For this review, take the finished solid that the model builds, in its own axes (mm). A direction names the side the tool comes from. Give positions to 0.01 mm unless a question says otherwise; leave off trailing zeros. Order: outer loops, then holes, each group sorted by start corner. A loop starts at its lowest first (then second) coordinate and runs counter-clockwise, first axis right, second up. Notation, with made-up numbers: (35.5, 32) -> (61.5, 32) arc R27 cw to (61.5, 49) -> close; hole circle Ø1 at (73.5, -25). An arc over 180 degrees is marked (long way). Return JSON: item names as keys, results as strings. Group by question number.
1) Insertion check: P1, Ø3.5, axis at x = -19.5, y = 8.5, coming from the +Z side (3 decimals); P2, Ø1, axis at x = 89.5, y = 2, coming from the -Z side (3 decimals); P3, Ø1, axis at y = 1.5, z = 42.5, coming from the +X side. Each pin has a flat end and moves straight along its axis. Give the tip position at first contact, or say it passes through.
2) Add section A-A (y = 6.25). Give the boundary of the cut face in (x, z) (3 decimals), then the cut area to 3 significant figures.
3) To check wall thickness, follow line 1 along Z through (x, y) = (-49, 6.75) (3 decimals); line 2 along Z through (x, y) = (65, 4.75) (3 decimals); line 3 along Z through (x, y) = (24.5, 7.75) (3 decimals). State the ranges of each line that lie inside material, in increasing order.
4) Add section C-C (z = 12.5). Give the boundary of the cut face in (x, y) (3 decimals).
5) Add section B-B (x = -17). Give the boundary of the cut face in (y, z) (3 decimals), then the cut area to 3 significant figures.
6) Add section D-D (x = 60.5). Give the boundary of the cut face in (y, z) (3 decimals), then the cut area to 3 significant figures.
7) For faces 1 (the face through (79.375, 6, -40)), 2 (the face through (-0.745, 7.727, -29.738)), 3 (the face through (82.55, 2, -43)), 4 (the face through (87, 2, 10.16)), list the 3-axis set-ups (+Z, -Z, +X, -X, +Y, -Y) from which the entire face can be reached by the end or side of a thin tool; tool diameter is ignored.
8) The part is to be moulded in two halves that separate along Z. For faces 5 (the face through (89, 2, 41.275)), 6 (the face through (1, 9.525, 40)), 7 (the face through (57.15, 9, 0)), say which applies: released by +Z, released by -Z, zero draft, split by the parting line, or undercut.
from build123d import *

# Parameters (mm, degrees)
SKETCH1_W           = 165.1
SKETCH1_H           = 88.9
BOSS_EXTRUDE1_DEPTH = 3.175
SKETCH3_W           = 82.55
SKETCH3_H           = 3.175
BOSS_EXTRUDE3_DEPTH = 12.7
SKETCH6_W           = 19.05
SKETCH6_H           = 3.175
CUT_EXTRUDE1_DEPTH  = 16.002
SKETCH8_W           = 154.94
SKETCH8_H           = 3.437080139
BOSS_EXTRUDE4_DEPTH = 6.35
SKETCH9_W           = 114.3
SKETCH9_H           = 69.85
BOSS_EXTRUDE5_DEPTH = 15.24
SKETCH12_W          = 88.9
SKETCH12_H          = 50.8
CUT_EXTRUDE2_DEPTH  = 15.24
CUT_EXTRUDE2_DRAFT  = 30


with BuildPart() as part:
    # Sketch1 → Boss-Extrude1 (new body)
    with BuildSketch(Plane(origin=(0, 0, 0), x_dir=(1, 0, 0), z_dir=(0, 1, 0))):
        Rectangle(SKETCH1_W, SKETCH1_H)
    extrude(amount=BOSS_EXTRUDE1_DEPTH)

    # Sketch3 → Boss-Extrude3 (add)
    with BuildSketch(Plane(origin=(82.55, 0, 0), x_dir=(0, 0, -1), z_dir=(1, 0, 0))):
        with Locations((0, 1.5875)):
            Rectangle(SKETCH3_W, SKETCH3_H)
    extrude(amount=BOSS_EXTRUDE3_DEPTH)

    # Sketch6 → Cut-Extrude1 (cut)
    with BuildSketch(Plane(origin=(95.25, 0, 0), x_dir=(0, 0, -1), z_dir=(1, 0, 0))):
        with Locations((-0.635, 1.5875)):
            Rectangle(SKETCH6_W, SKETCH6_H)
    extrude(amount=-CUT_EXTRUDE1_DEPTH, mode=Mode.SUBTRACT)

    # Sketch8 → Boss-Extrude4 (add)
    with BuildSketch(Plane(origin=(0, 3.175, 0), x_dir=(1, 0, 0), z_dir=(0, 1, 0))):
        with Locations((1.905, -39.556459931)):
            Rectangle(SKETCH8_W, SKETCH8_H)
        with Locations((1.905, 39.556459931)):
            Rectangle(SKETCH8_W, SKETCH8_H)
    extrude(amount=BOSS_EXTRUDE4_DEPTH)

    # Sketch9 → Boss-Extrude5 (add)
    with BuildSketch(Plane(origin=(0, 0, 0), x_dir=(1, 0, 0), z_dir=(0, 1, 0))):
        Rectangle(SKETCH9_W, SKETCH9_H)
    extrude(amount=BOSS_EXTRUDE5_DEPTH)


with BuildPart() as cut_extrude2_tool:
    # Sketch12 → Cut-Extrude2 (with draft: the straight prism first)
    with BuildSketch(Plane(origin=(0, 15.24, 0), x_dir=(1, 0, 0), z_dir=(0, 1, 0))):
        Rectangle(SKETCH12_W, SKETCH12_H)
    extrude(amount=-CUT_EXTRUDE2_DEPTH)
    # Cut-Extrude2: the draft: its side faces are tilted about the plane it starts from
    cut_extrude2_sides = [cut_extrude2_tool.faces().sort_by_distance(p)[0] for p in [
        (-44.45, 7.62, 0),
        (0, 7.62, 25.4),
        (44.45, 7.62, 0),
        (0, 7.62, -25.4),
    ]]
    draft(cut_extrude2_sides, Plane(origin=(0, 15.24, 0), x_dir=(1, 0, 0), z_dir=(0, 1, 0)), CUT_EXTRUDE2_DRAFT)


with BuildPart() as part_1:
    add(part.part)

    # Cut-Extrude2: cut by cut_extrude2_tool
    add(cut_extrude2_tool.part, mode=Mode.SUBTRACT)


solid = part_1.part
Evaluation:
{
 "1": {"P1": "z = 41.275", "P2": "z = -41.275", "P3": "x = 82.55"},
 "2": {"outline": "(-75.565, -41.275) -> (79.375, -41.275) -> (79.375, -37.838) -> (-75.565, -37.838) -> close; (-75.565, 37.838) -> (79.375, 37.838) -> (79.375, 41.275) -> (-75.565, 41.275) -> close; (-57.15, -34.925) -> (57.15, -34.925) -> (57.15, 34.925) -> (-57.15, 34.925) -> close; hole (-49.64, -30.59) -> (49.64, -30.59) -> (49.64, 30.59) -> (-49.64, 30.59) -> close", "area": "2,970 mm^2"},
 "3": {"line 1": "-41.275 to -37.838, -34.925 to -30.302, 30.302 to 34.925, 37.838 to 41.275", "line 2": "-41.275 to -37.838, 37.838 to 41.275", "line 3": "-41.275 to -37.838, -34.925 to -29.724, 29.724 to 34.925, 37.838 to 41.275"},
 "4": {"outline": "(-82.55, 0) -> (-53.249, 0) -> (-44.45, 15.24) -> (-57.15, 15.24) -> (-57.15, 3.175) -> (-82.55, 3.175) -> close; (44.45, 15.24) -> (53.249, 0) -> (95.25, 0) -> (95.25, 3.175) -> (57.15, 3.175) -> (57.15, 15.24) -> close"},
 "5": {"outline": "(0, -44.45) -> (3.175, -44.45) -> (3.175, -41.275) -> (9.525, -41.275) -> (9.525, -37.838) -> (3.175, -37.838) -> (3.175, -34.925) -> (15.24, -34.925) -> (15.24, -25.4) -> (0, -34.199) -> close; (0, 34.199) -> (15.24, 25.4) -> (15.24, 34.925) -> (3.175, 34.925) -> (3.175, 37.838) -> (9.525, 37.838) -> (9.525, 41.275) -> (3.175, 41.275) -> (3.175, 44.45) -> (0, 44.45) -> close", "area": "260 mm^2"},
 "6": {"outline": "(0, -44.45) -> (3.175, -44.45) -> (3.175, -41.275) -> (9.525, -41.275) -> (9.525, -37.838) -> (3.175, -37.838) -> (3.175, 37.838) -> (9.525, 37.838) -> (9.525, 41.275) -> (3.175, 41.275) -> (3.175, 44.45) -> (0, 44.45) -> close", "area": "326 mm^2"},
 "7": {"face 1": "+Z, -Z, +X, +Y", "face 2": "-Y", "face 3": "-Z, +X, +Y, -Y", "face 4": "+X, +Y, -Y"},
 "8": {"face 5": "released by +Z", "face 6": "zero draft", "face 7": "undercut"}
}
